```python
from build123d import *

# Parameters (mm, degrees)
EXTRUDE_THIN1_DEPTH = 35
BOSS_EXTRUDE2_DEPTH = 10
SKETCH4_R           = 9
CUT_EXTRUDE1_DEPTH  = 279.07373123
CIRPATTERN1_COUNT   = 4


with BuildPart() as part:
    # Sketch2 → Extrude-Thin1 (new, symmetric)
    with BuildSketch(Plane.XY):
        Polygon((-200, 0), (0, 0), (0, -200), (-10, -200), (-10, -10), (-200, -10), align=None)
    extrude(amount=EXTRUDE_THIN1_DEPTH, both=True)

    # Sketch3 → Boss-Extrude2 (add)
    with BuildSketch(Plane(origin=(0, 0, -30), x_dir=(-1, 0, 0), z_dir=(0, 0, -1))):
        with BuildLine():
            Line((30, -10), (10, -30))
            Line((10, -30), (10, -185))
            ThreePointArc((10, -185), (67.181073979, -67.181073979), (185, -10))
            Line((185, -10), (30, -10))
        make_face()
    boss_extrude2 = extrude(amount=-BOSS_EXTRUDE2_DEPTH)

    # Mirror1: Boss-Extrude2 across plane
    add(boss_extrude2.mirror(Plane.XY))

    # Sketch4 → Cut-Extrude1 (cut, through all)
    with BuildSketch(Plane.ZY.offset(10)):
        with Locations(Location((0, -55, 0), (0, 0, 270))):
            Circle(SKETCH4_R)
        with Locations(Location((0, -175, 0), (0, 0, 270))):
            Circle(SKETCH4_R)
    cut_extrude1 = extrude(amount=-CUT_EXTRUDE1_DEPTH, mode=Mode.SUBTRACT)

    # CirPattern1: Cut-Extrude1 ×4 about axis
    cirpattern1_axis = Axis((0, 0, 35), (0, 0, -1))
    for i in range(1, CIRPATTERN1_COUNT):
        add(cut_extrude1.rotate(cirpattern1_axis, i * 360 / CIRPATTERN1_COUNT), mode=Mode.SUBTRACT)


solid = part.part
```
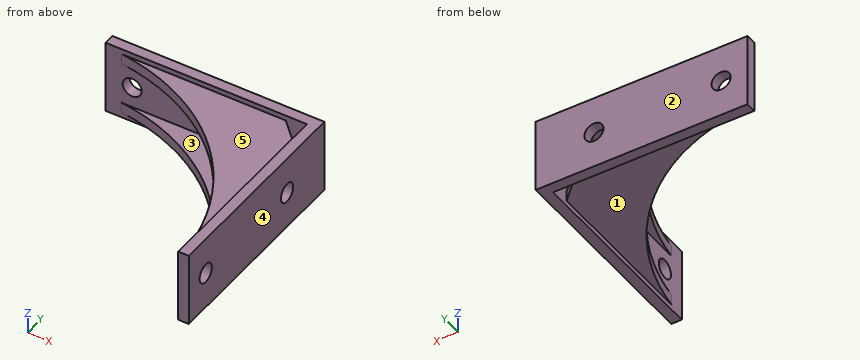
Geometry: final body of the model. Coordinates: model frame, mm. Face numbers are marked on the shaded views. A direction names the side the tool comes from. Coordinates: 2 decimals unless noted, no trailing zeros. Write each loop counter-clockwise with the first axis right and the second up, starting at its lowest first coordinate (ties: lowest second). Pieces come first, ordered by that corner, then holes. Notation, with made-up numbers: M 42,19.5 L 66,19.5 A17 ccw 66,44.5 Z; hole C 53.25,2.5 d2. An arc over 180 degrees is marked long. Use CSV: the item, a comma, the result in double quotes. Start each with the question number.
1. Mould query, pull axis Z, two halves, no side actions, for the marked faces 1, 2 and 3. Classes: pulls with the +Z half, pulls with the -Z half, needs draft (parallel to the pull), parting line crosses it, or undercut.
2. Reachability of the marked faces 4 and 5 from +Z, -Z, +X, -X, +Y, -Y: full face, straight path, thin tool, end or side. Return the list, or none.
3. Cut plane B-B on y = -18. Return the cut outline in (x, z), plus the area to 3 significant figures.
4. Ray query, probe 1 along Z at (x, y) = (-104, -11); probe 2 along Z at (x, y) = (-4.5, -55); probe 3 along X at (y, z) = (-21, 4.5). Return the intervals inside material, ascending.
5. First-contact query: P1, Ø14.5, axis at y = -55, z = 0, coming from the +X side; P2, Ø2, axis at y = -48, z = -14.5, coming from the -X side. Flat tips, straight axial feed; report the tip coordinate or a pass-through.
6. Cut plane C-C on x = -175. Return the cut outline in (y, z).
7. Cut plane A-A on z = 0. Return the cut outline in (x, y).
Entries:
1,face 1,"pulls with the -Z half"
1,face 2,"needs draft"
1,face 3,"undercut"
2,face 4,"+Z, -Z, +X, +Y, -Y"
2,face 5,"+Z, -X, -Y"
3,outline,"M -148.02,-30 L -22,-30 L -22,-20 L -148.02,-20 Z; M -148.02,20 L -22,20 L -22,30 L -148.02,30 Z; M -10,-35 L 0,-35 L 0,35 L -10,35 Z"
3,area,"3,220 mm²"
4,probe 1,"-30 to -20, 20 to 30"
4,probe 2,"-35 to -9, 9 to 35"
4,probe 3,"-10 to 0"
5,P1,"through"
5,P2,"x = -10"
6,outline,"M -11.45,-30 L -10,-30 L -10,-35 L 0,-35 L 0,-9 L -10,-9 L -10,-20 L -11.45,-20 Z; M -11.45,20 L -10,20 L -10,9 L 0,9 L 0,35 L -10,35 L -10,30 L -11.45,30 Z"
7,outline,"M -200,-10 L -184,-10 L -184,0 L -200,0 Z; M -166,-10 L -64,-10 L -64,0 L -166,0 Z; M -46,-10 L -10,-10 L -10,-46 L 0,-46 L 0,0 L -46,0 Z; M -10,-200 L 0,-200 L 0,-184 L -10,-184 Z; M -10,-166 L 0,-166 L 0,-64 L -10,-64 Z"
